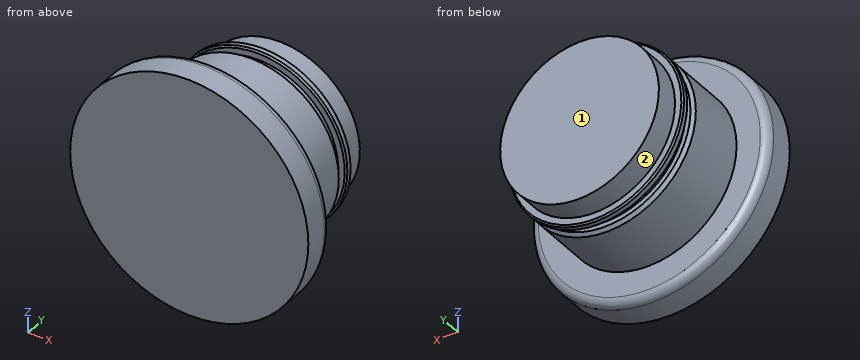
```python
from build123d import *

# Parameters (mm, degrees)
SKETCH2_R           = 75
BOSS_EXTRUDE1_DEPTH = 20
FILLET1_R           = 5
SKETCH6_R           = 55
BOSS_EXTRUDE4_DEPTH = 40
SKETCH7_R           = 50
BOSS_EXTRUDE5_DEPTH = 5
SKETCH8_R           = 55
BOSS_EXTRUDE7_DEPTH = 5
SKETCH10_R          = 50
BOSS_EXTRUDE8_DEPTH = 15
CHAMFER7_SIZE       = 1
CHAMFER8_SIZE       = 2


with BuildPart() as part:
    # Sketch2 → Boss-Extrude1 (new body)
    with BuildSketch(Plane(origin=(0, 0, 0), x_dir=(1, 0, 0), z_dir=(0, 1, 0))):
        with Locations(Location((0, 0, 0), (0, 0, 270))):
            Circle(SKETCH2_R)
    extrude(amount=BOSS_EXTRUDE1_DEPTH)

    # Fillet1
    fillet1_edges = [part.edges().sort_by_distance(p)[0] for p in [
        (0, 20, -75),
    ]]
    fillet(fillet1_edges, radius=FILLET1_R)

    # Sketch6 → Boss-Extrude4 (add)
    with BuildSketch(Plane(origin=(0, 20, 0), x_dir=(1, 0, 0), z_dir=(0, 1, 0))):
        with Locations(Location((0, 0, 0), (0, 0, 270))):
            Circle(SKETCH6_R)
    extrude(amount=BOSS_EXTRUDE4_DEPTH)

    # Sketch7 → Boss-Extrude5 (add)
    with BuildSketch(Plane(origin=(0, 60, 0), x_dir=(1, 0, 0), z_dir=(0, 1, 0))):
        with Locations(Location((0, 0, 0), (0, 0, 270))):
            Circle(SKETCH7_R)
    extrude(amount=BOSS_EXTRUDE5_DEPTH)

    # Sketch8 → Boss-Extrude7 (add)
    with BuildSketch(Plane(origin=(0, 65, 0), x_dir=(1, 0, 0), z_dir=(0, 1, 0))):
        with Locations(Location((0, 0, 0), (0, 0, 270))):
            Circle(SKETCH8_R)
    extrude(amount=BOSS_EXTRUDE7_DEPTH)

    # Sketch10 → Boss-Extrude8 (add)
    with BuildSketch(Plane(origin=(0, 70, 0), x_dir=(1, 0, 0), z_dir=(0, 1, 0))):
        with Locations(Location((0, 0, 0), (0, 0, 270))):
            Circle(SKETCH10_R)
    extrude(amount=BOSS_EXTRUDE8_DEPTH)

    # Chamfer7
    chamfer7_edges = [part.edges().sort_by_distance(p)[0] for p in [
        (0, 65, -55),
        (0, 70, -55),
    ]]
    chamfer(chamfer7_edges, length=CHAMFER7_SIZE)

    # Chamfer8
    chamfer8_edges = [part.edges().sort_by_distance(p)[0] for p in [
        (0, 60, -55),
    ]]
    chamfer(chamfer8_edges, length=CHAMFER8_SIZE)


solid = part.part
```
The listing builds one solid part. Answer for the finished solid, in the listing's coordinates (mm). Face numbers are marked on the shaded views. A direction names the side the tool comes from. Coordinates: 2 decimals unless noted, no trailing zeros. Loops run counter-clockwise (first coordinate to the right, second up) from the corner with the lowest first, then second, coordinate; pieces in that order, holes last. Notation, with made-up numbers: (55.5, -33) -> (80.5, -33) arc R22 ccw to (80.5, -9) -> close; hole circle Ø2 at (76.5, 2.5). An arc over 180 degrees is marked (long way). Use one line per item in the form item = value. Start each with the question number.
Item 1: The part is cut by section B-B on y = 24.5. Determine the outline of the cut face in (x, z).
Item 2: The part is cut by section A-A on z = 0. Determine the outline of the cut face in (x, y).
Item 3: Consider L1, parallel to X at y = 58.5, z = -12.5; L2, parallel to Y at x = 47, z = -35; L3, parallel to Z at x = -15.5, y = 78.5. Determine where each line is inside the solid, lowest interval first. Write a range as [from, to].
Item 4: The part is cut by section C-C on y = 74.5. Determine the outline of the cut face in (x, z).
Item 5: Flat-ended cylindrical pins translate along their axes: pin 1 Ø4 at (y, z) = (66.5, 26.5) entering from -X; pin 2 Ø8 at (x, y) = (13.5, 47.5) entering from +Z; pin 3 Ø6 at (x, z) = (-57, 24.5) entering from +Y. Find the tip coordinate at first contact, or state that the pin passes through.
Item 6: A tool of negligible diameter and unlimited length cuts with its end or side. For the marked faces 1 and 2, from which of +Z, -Z, +X, -X, +Y, -Y can it reach the whole face along a straight path? Write none if from no direction.
Answer key:
q1.outline = circle Ø110 at (0, 0)
q2.outline = (-75, 0) -> (75, 0) -> (75, 15) arc R5 ccw to (70, 20) -> (55, 20) -> (55, 58) -> (53, 60) -> (50, 60) -> (50, 65) -> (54, 65) -> (55, 66) -> (55, 69) -> (54, 70) -> (50, 70) -> (50, 85) -> (-50, 85) -> (-50, 70) -> (-54, 70) -> (-55, 69) -> (-55, 66) -> (-54, 65) -> (-50, 65) -> (-50, 60) -> (-53, 60) -> (-55, 58) -> (-55, 20) -> (-70, 20) arc R5 ccw to (-75, 15) -> close
q3.L1 = [-53.05, 53.05]
q3.L2 = [0, 20]
q3.L3 = [-47.54, 47.54]
q4.outline = circle Ø100 at (0, 0)
q5.pin_1 = -49.24
q5.pin_2 = 54.17
q5.pin_3 = 20
q6.face_1 = +Z, -Z, +X, -X, +Y
q6.face_2 = +Y
